Verification items for the finished model (mm, model axes). Face numbers are marked on the shaded views. Round coordinates to 2 decimals unless told otherwise and drop trailing zeros. Order: outer loops, then holes, each group sorted by start corner. A loop starts at its lowest first (then second) coordinate and runs counter-clockwise, first axis right, second up.
```python
from build123d import *

# Parameters (mm, degrees)
F0_R     = 10
F1_DEPTH = 10
F2_R     = 7.4
F3_DEPTH = 4.6
F4_R     = 5
F5_R     = 1


with BuildPart() as f1:
    # F0 (on Top) → F1 (new body)
    with BuildSketch(Plane.XY):
        Circle(F0_R)
    extrude(amount=F1_DEPTH)

    # F2 (on face) → F3 (cut)
    with BuildSketch(Plane.XY.offset(10)):
        Circle(F2_R)
    extrude(amount=-F3_DEPTH, mode=Mode.SUBTRACT)

    # F4
    f4_edges = [f1.edges().sort_by_distance(p)[0] for p in [
        (-10, 0, 0),
    ]]
    fillet(f4_edges, radius=F4_R)

    # F5
    f5_edges = [f1.edges().sort_by_distance(p)[0] for p in [
        (-7.4, 0, 10),
        (-10, 0, 10),
    ]]
    fillet(f5_edges, radius=F5_R)


solid = f1.part
```
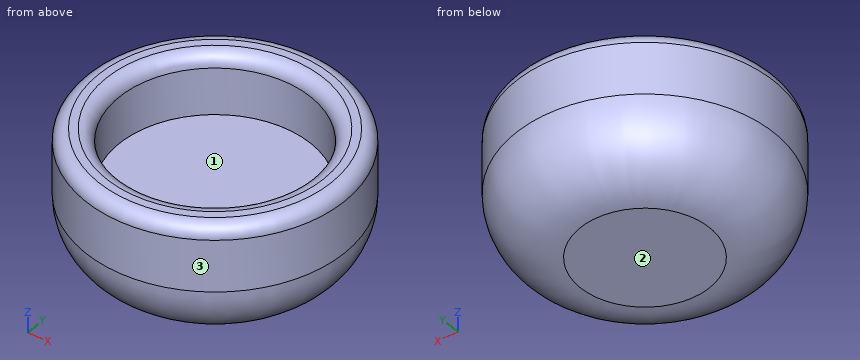
1) Go/stop test with flat-tipped pins: pin 1 Ø2 at (y, z) = (-7, 1) entering from -X; pin 2 Ø5 at (x, z) = (-5.5, 2.5) entering from -Y; pin 3 Ø1.5 at (x, z) = (2.5, 2) entering from +Y. Record where each tip stops, or that it passes through.
2) Draft check along X on the marked faces 1, 2 and 3. Enter one of: released by +X, released by -X, zero draft, split by the parting line, or undercut.
3) Sectioned sample at A-A on z = 6.25. Record the cut outline in (x, y), then the cut area to 3 significant figures.
4) Scan lines: probe 1 along Y at (x, z) = (0, 8.2); probe 2 along Z at (x, y) = (2, -1.75); probe 3 along Y at (x, z) = (-3, 9.75). Record each from-to range of solid material in increasing order.
5) Sectioned sample at B-B on z = 9.25. Record the cut outline in (x, y).
Returned:
1. pin 1: stops at x = -6.1
1. pin 2: stops at y = -9.26
1. pin 3: stops at y = 9.17
2. face 1: undercut
2. face 2: zero draft
2. face 3: split by the parting line
3. outline: circle Ø20 at (0, 0); hole circle Ø14.8 at (0, 0)
3. area: 142 mm2
4. probe 1: y = -10 to -7.4, 7.4 to 10
4. probe 2: z = 0 to 5.4
4. probe 3: y = -9.18 to -7.13, 7.13 to 9.18
5. outline: circle Ø19.94 at (0, 0); hole circle Ø14.86 at (0, 0)
